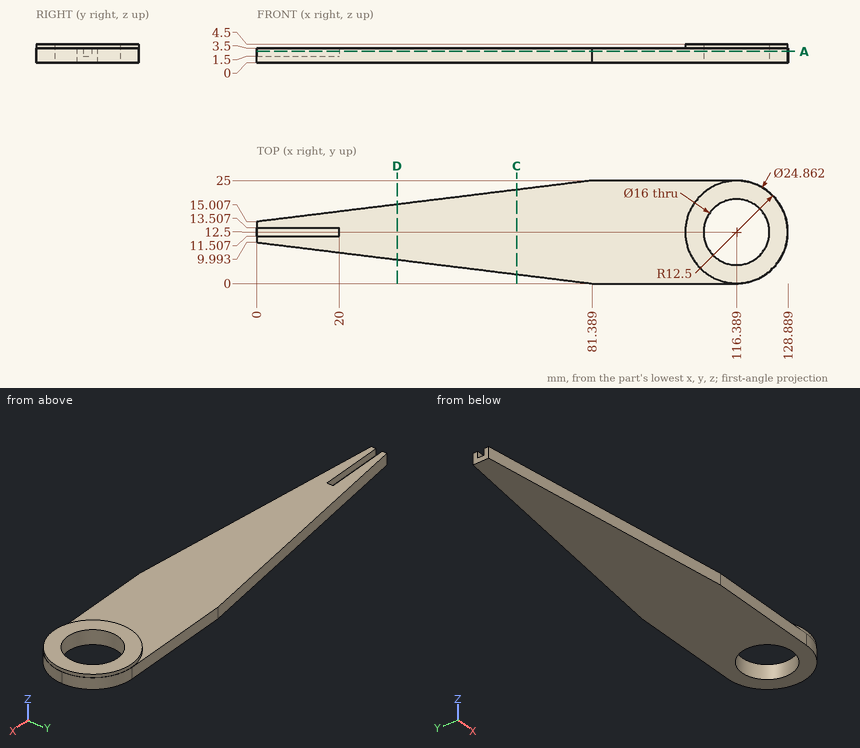
Geometry check sheet. Reference: drawing and pictorial views, mm from the part's lowest x, y, z. Round coordinates to 2 decimals unless told otherwise and drop trailing zeros. Write each loop counter-clockwise with the first axis right and the second up, starting at its lowest first coordinate (ties: lowest second). Pieces come first, ordered by that corner, then holes.
(1) Depth check by flat-ended pin: pin 1 Ø1.6 at (x, y) = (10, 12.5) entering from +Z; pin 2 Ø6 at (x, y) = (88.5, 10) entering from +Z; pin 3 Ø2 at (x, z) = (36, 4) entering from +Y. Enter the tip coordinate at first touch or a pass-through.
Returned:
pin 1: stops at z = 1.5
pin 2: stops at z = 3.5
pin 3: stops at y = 19.53
(2) Section check D-D (x = 34). Enter the section's corners in (y, z), plus the area to 3 significant figures.
Returned:
outline: (5.82, 0) - (19.18, 0) - (19.18, 3.5) - (5.82, 3.5) - close
area: 46.8 mm2
(3) Section check A-A (z = 2.7). Enter the section's corners in (x, y), plus the area to 3 significant figures.
Returned:
outline: (0, 9.99) - (81.39, 0) - (116.39, 0) arc R12.5 ccw to (128.89, 12.5) arc R12.5 ccw to (116.39, 25) - (81.39, 25) - (0, 15.01) - (0, 13.51) - (20, 13.51) - (20, 11.51) - (0, 11.51) - close; hole circle Ø16 at (116.39, 12.5)
area: 2,100 mm2
(4) Section check C-C (x = 63). Enter the section's corners in (y, z).
Returned:
outline: (2.26, 0) - (22.74, 0) - (22.74, 3.5) - (2.26, 3.5) - close
(5) Material ranges on line 1 (X direction, y = 12, z = 0.95) (1 decimal); line 2 (X direction, y = 13, z = 2.4) (1 decimal); line 3 (Z direction, x = 90, y = 11.5), recorded low to high.
Returned:
line 1: x = 0 to 108.4, 124.4 to 128.9
line 2: x = 20 to 108.4, 124.4 to 128.9
line 3: z = 0 to 3.5
